Verification items for this drawing (mm, ordinates from the low corner). Give positions to 0.01 mm unless a question says otherwise; leave off trailing zeros. Order: outer loops, then holes, each group sorted by start corner. A loop starts at its lowest first (then second) coordinate and runs counter-clockwise, first axis right, second up. Notation, with made-up numbers: M -31.5,22.5 L 27.5,22.5 A34 cw 27.5,55.5 Z; hole C 79.25,-20 d2. An arc over 180 degrees is marked long. Answer as a JSON object with one key per item and string values.
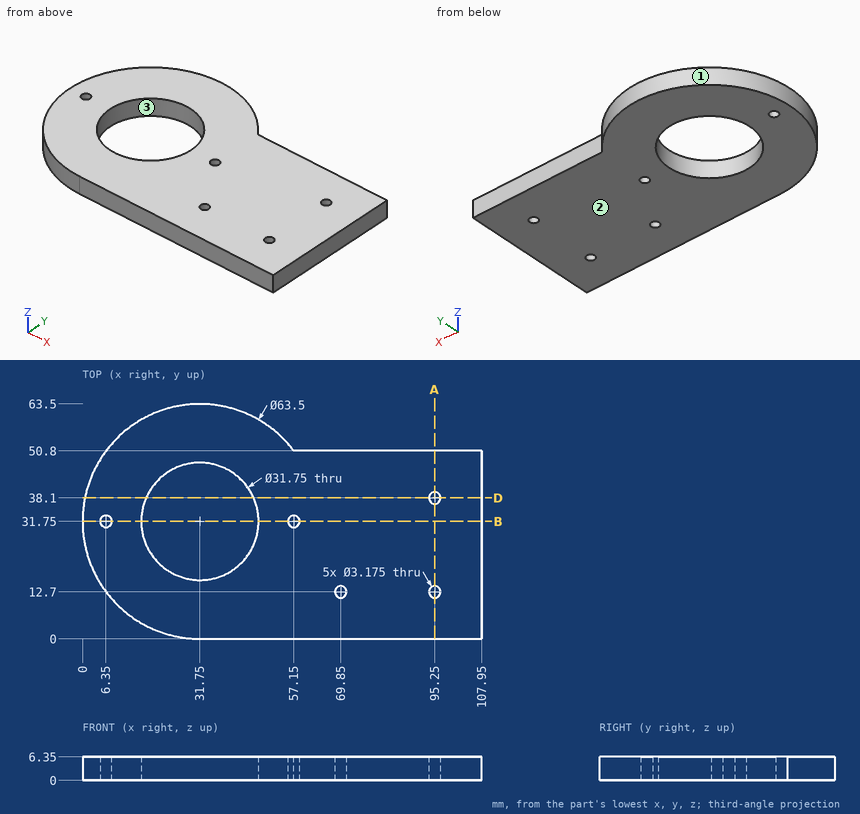
Q1. Gauge pin test, flat ends, axial feed: pin 1 Ø3 at (x, z) = (91, 2.5) entering from +Y; pin 2 Ø2.5 at (x, y) = (95.25, 12.7) entering from +Z. Record the tip position at first contact, or that the pin passes through.
Resolved:
{"pin 1": "stops at y = 50.8", "pin 2": "passes through"}
Q2. Section check B-B on y = 31.75. Count the separate pieces of the cut face and the enclosed holes in it, then the cut area to 3 significant figures.
Resolved:
{"separate pieces": "4", "enclosed holes": "0", "area": "444 mm²"}
Q3. Release check for a two-part mould opening along X. For the marked faces 1, 2 and 3 record: +X half, -X half, draft (parallel to the pull), parting line (faces both ways), or undercut.
Resolved:
{"face 1": "parting line", "face 2": "draft", "face 3": "undercut"}
Q4. Section check A-A on x = 95.25. Record the cut outline in (y, z).
Resolved:
{"outline": "M 0,0 L 11.11,0 L 11.11,6.35 L 0,6.35 Z; M 14.29,0 L 36.51,0 L 36.51,6.35 L 14.29,6.35 Z; M 39.69,0 L 50.8,0 L 50.8,6.35 L 39.69,6.35 Z"}
Q5. Section check D-D on y = 38.1. Record the cut outline in (x, z), then the cut area to 3 significant figures.
Resolved:
{"outline": "M 0.64,0 L 17.2,0 L 17.2,6.35 L 0.64,6.35 Z; M 46.3,0 L 93.66,0 L 93.66,6.35 L 46.3,6.35 Z; M 96.84,0 L 107.95,0 L 107.95,6.35 L 96.84,6.35 Z", "area": "476 mm²"}
Q6. Material ranges on L1, parallel to Y at x = 95.25, z = 2; L2, parallel to Y at x = 57.15, z = 4.75; L3, parallel to Y at x = 31.75, z = 3.75 (3 decimals), recorded low to high.
Resolved:
{"L1": "y = 0 to 11.11, 14.29 to 36.51, 39.69 to 50.8", "L2": "y = 0 to 30.16, 33.34 to 50.8", "L3": "y = 0 to 15.875, 47.625 to 63.5"}
